Work out the finished part from the listing and answer in its coordinate system (mm). Round coordinates to 2 decimals unless told otherwise and drop trailing zeros. Loops run counter-clockwise (first coordinate to the right, second up) from the corner with the lowest first, then second, coordinate; pieces in that order, holes last. Notation, with made-up numbers: (5.5, 52.25) -> (31.5, 52.25) arc R25 cw to (31.5, 67.25) -> close; hole circle Ø8 at (51.25, 50.5). An arc over 180 degrees is marked (long way). Write item = value, one per line. Start each with the question number.
```python
from build123d import *

# Parameters (mm, degrees)
SKETCH1_R           = 2
SKETCH1_R_2         = 2.5
BOSS_EXTRUDE1_DEPTH = 5
SKETCH8_R           = 3
BOSS_EXTRUDE3_DEPTH = 10


with BuildPart() as part:
    # Sketch1 → Boss-Extrude1 (new body)
    with BuildSketch(Plane(origin=(0, 0, 0), x_dir=(0.498528904, -0.866873077, 0), z_dir=(0, 0, 1))):
        with BuildLine():
            Line((8.899126574, 3.869128256), (-2.35642803, 24.179978159))
            ThreePointArc((-2.35642803, 24.179978159), (-9.345167797, 25.255857552), (-10.421047189, 18.267117784))
            Line((-10.421047189, 18.267117784), (1.120951981, -3.909046337))
            ThreePointArc((1.120951981, -3.909046337), (8.899126574, -3.909046337), (8.899126574, 3.869128256))
        make_face()
        with Locations((-6.38873761, 21.223547972)):
            Circle(SKETCH1_R, mode=Mode.SUBTRACT)
        with Locations((5.010039278, -0.019959041)):
            Circle(SKETCH1_R_2, mode=Mode.SUBTRACT)
        with BuildLine():
            Line((8.899126574, -46.838046337), (8.899126574, -3.909046337))
            ThreePointArc((8.899126574, -3.909046337), (5.010039278, -5.519959041), (1.120951981, -3.909046337))
            Line((1.120951981, -3.909046337), (0.353553391, -2.434608777))
            Line((0.353553391, -2.434608777), (0.353553391, -46.838046337))
            Line((0.353553391, -46.838046337), (8.899126574, -46.838046337))
        make_face()
    extrude(amount=BOSS_EXTRUDE1_DEPTH)

    # Sketch8 → Boss-Extrude3 (add)
    with BuildSketch(Plane(origin=(0, 0, 0), x_dir=(-1, 0, 0), z_dir=(0, 0, -1))):
        with Locations((25.293181008, -19.882635909)):
            Circle(SKETCH8_R)
    extrude(amount=BOSS_EXTRUDE3_DEPTH)

    # Sketch9 → Cut-Revolve1 (revolve, cut)
    with BuildSketch(Plane(origin=(2.306364199, -4.010449578, 0), x_dir=(-0.866873077, -0.498528904, 0), z_dir=(0.498528904, -0.866873077, 0))):
        with BuildLine():
            Line((32.838046337, 10), (34.838046337, 10))
            Line((34.838046337, 10), (34.838046337, 7))
            ThreePointArc((34.838046337, 7), (34.292209794, 8.802775638), (32.838046337, 10))
        make_face()
    revolve(axis=Axis((-25.293181008, -19.882635909, -10), (0, 0, 1)), mode=Mode.SUBTRACT)


solid = part.part
```
Item 1: Section B-B (y = -4) is taken. Determine the outline of the cut face in (x, z).
Item 2: Find the intervals of material crossed by line 1 along Z through (x, y) = (-14.5, -13); line 2 along Y through (x, z) = (-6.5, 4); line 3 along Y through (x, z) = (-23.5, 1.25), in increasing order. Write a range as [from, to].
Item 3: Section C-C (y = -24.5) is taken. Determine the outline of the cut face in (x, z).
Item 4: The mould has two halves that part along X. Classify faces 1 (the cylindrical face through (15.65, 18.07, 2.46)), 2 (the cylindrical face through (-28.064, -21.032, -3.451)), 3 (the flat face through (-38.326, -27.309, 2.465)): pulls with the +X half, pulls with the -X half, needs draft (parallel to the pull), parting line crosses it, or undercut.
Item 5: Section A-A (x = 2) is taken. Determine the outline of the cut face in (y, z).
Item 6: Section D-D (x = 9.5) is taken. Determine the outline of the cut face in (y, z).
Item 7: Flat-ended cylindrical pins translate along their axes: pin 1 (12 mm diameter, centred on x = -6, y = -25, fed in from +Z); pin 2 (15.5 mm diameter, centred on x = -1.5, y = 5, fed in from -Z); pin 3 (8 mm diameter, centred on y = -14, z = 0.5, fed in from +X). Find the tip coordinate at first contact, or state that the pin passes through.
Worked answers:
q1.outline = (-6.25, 0) -> (0.01, 0) -> (0.01, 5) -> (-6.25, 5) -> close; (4.96, 0) -> (8.87, 0) -> (8.87, 5) -> (4.96, 5) -> close
q2.line_1 = [0, 5]
q2.line_2 = [-14, -4.15]
q2.line_3 = [-23.78, -13.92]
q3.outline = (-39.94, 0) -> (-24.75, 0) -> (-24.75, 5) -> (-39.94, 5) -> close
q4.face_1 = undercut
q4.face_2 = parting line crosses it
q4.face_3 = pulls with the -X half
q5.outline = (-9.83, 0) -> (-6.81, 0) -> (-6.81, 5) -> (-9.83, 5) -> close; (-1.9, 0) -> (4.63, 0) -> (4.63, 5) -> (-1.9, 5) -> close
q6.outline = (-2.95, 0) -> (16.36, 0) -> (16.36, 5) -> (-2.95, 5) -> close
q7.pin_1 = through
q7.pin_2 = 0
q7.pin_3 = 0.46
